Could you check a few things on this model? Use its own coordinates, in mm. Face numbers are marked on the shaded views. A direction names the side the tool comes from. Round coordinates to 2 decimals unless told otherwise and drop trailing zeros. Write each loop counter-clockwise with the first axis right and the second up, starting at its lowest first coordinate (ties: lowest second). Pieces come first, ordered by that corner, then holes. Notation, with made-up numbers: (62, 66) -> (121, 66) arc R35 ccw to (121, 101) -> close; hole circle Ø1 at (-29, -9.5). An arc over 180 degrees is marked (long way). Return JSON: item names as keys, results as strings.
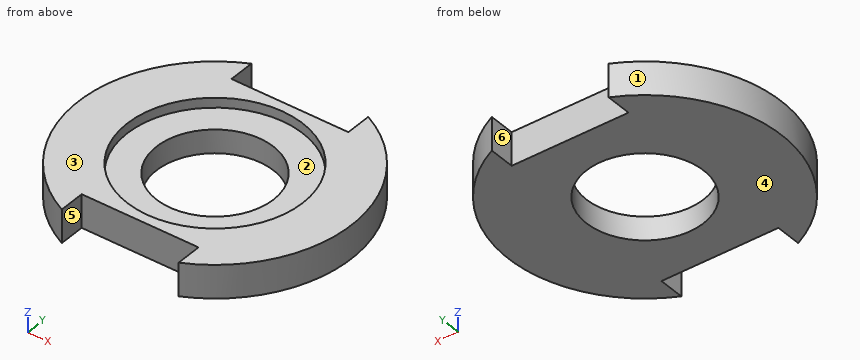
from build123d import *

# Parameters (mm, degrees)
SKETCH_1_R          = 14
EXTRUDE_1_DEPTH     = 3.4
SKETCH_2_R          = 6
CUT_EXTRUDE_1_DEPTH = 3.4
SKETCH_3_W          = 12
SKETCH_3_H          = 8
CUT_EXTRUDE_2_DEPTH = 3.4
SKETCH_4_R          = 9
CUT_EXTRUDE_3_DEPTH = 1


with BuildPart() as part:
    # 스케치1 → 보스-돌출1 (new body)
    with BuildSketch(Plane.XY):
        Circle(SKETCH_1_R)
    extrude(amount=EXTRUDE_1_DEPTH)

    # 스케치2 → 컷-돌출1 (cut)
    with BuildSketch(Plane.XY.offset(3.4)):
        Circle(SKETCH_2_R)
    extrude(amount=-CUT_EXTRUDE_1_DEPTH, mode=Mode.SUBTRACT)

    # 스케치3 → 컷-돌출2 (cut)
    with BuildSketch(Plane.XY.offset(3.4)):
        with Locations((0, 14)):
            Rectangle(SKETCH_3_W, SKETCH_3_H)
        with Locations((0, -14)):
            Rectangle(SKETCH_3_W, SKETCH_3_H)
    extrude(amount=-CUT_EXTRUDE_2_DEPTH, mode=Mode.SUBTRACT)

    # 스케치4 → 컷-돌출3 (cut)
    with BuildSketch(Plane.XY.offset(3.4)):
        Circle(SKETCH_4_R)
    extrude(amount=-CUT_EXTRUDE_3_DEPTH, mode=Mode.SUBTRACT)


solid = part.part
1) If I drill on probe 1 along Y at (x, z) = (0, 1.05); probe 2 along Y at (x, z) = (0, 2.9); probe 3 along Z at (x, y) = (-5.75, -5.75), over which ranges is the centre line in solid material (lowest first)? Write a range as [from, to].
Return value:
{"probe 1": "[-10, -6], [6, 10]", "probe 2": "[-10, -9], [9, 10]", "probe 3": "[0, 2.4]"}
2) I want a section at A-A, the plane x = 0. Please give me the cut outline in (y, z), and give its area (3 significant figures).
Return value:
{"outline": "(-10, 0) -> (-6, 0) -> (-6, 2.4) -> (-9, 2.4) -> (-9, 3.4) -> (-10, 3.4) -> close; (6, 0) -> (10, 0) -> (10, 3.4) -> (9, 3.4) -> (9, 2.4) -> (6, 2.4) -> close", "area": "21.2 mm²"}
3) I want a section at D-D, the plane y = -7. Please give me the cut outline in (x, z).
Return value:
{"outline": "(-12.12, 0) -> (12.12, 0) -> (12.12, 3.4) -> (5.66, 3.4) -> (5.66, 2.4) -> (-5.66, 2.4) -> (-5.66, 3.4) -> (-12.12, 3.4) -> close"}
4) I want a section at B-B, the plane z = 2.95. Please give me the cut outline in (x, y), and give its area (3 significant figures).
Return value:
{"outline": "(-6, -12.65) -> (-6, -10) -> (6, -10) -> (6, -12.65) arc R14 ccw to (6, 12.65) -> (6, 10) -> (-6, 10) -> (-6, 12.65) arc R14 ccw to start; hole circle Ø18 at (0, 0)", "area": "276 mm²"}
5) I want a section at C-C, the plane y = 0. Please give me the cut outline in (x, z), and give its area (3 significant figures).
Return value:
{"outline": "(-14, 0) -> (-6, 0) -> (-6, 2.4) -> (-9, 2.4) -> (-9, 3.4) -> (-14, 3.4) -> close; (6, 0) -> (14, 0) -> (14, 3.4) -> (9, 3.4) -> (9, 2.4) -> (6, 2.4) -> close", "area": "48.4 mm²"}
6) For the marked faces 4, 5 and 6, which set-ups out of +Z, -Z, +X, -X, +Y, -Y let a thin tool reach every point of the face, with its end or its side?
Return value:
{"face 4": "-Z, +X, -X, +Y, -Y", "face 5": "+Z, -Z, -Y", "face 6": "+Z, -Z, +Y"}
7) Thinking about a two-plate mould opening in Y: for the marked faces 1, 2 and 3, which applies, pulls with the +Y half, pulls with the -Y half, needs draft (parallel to the pull), parting line crosses it, or undercut?
Return value:
{"face 1": "parting line crosses it", "face 2": "undercut", "face 3": "needs draft"}
8) Will these pins go through, and if not, where does the flat tip stop? pin 1 Ø1.3 at (y, z) = (-10.5, 1.5) entering from -X; pin 2 Ø7 at (x, y) = (0, 0) entering from +Z; pin 3 Ø1 at (x, z) = (-7, 1.5) entering from -Y; pin 4 Ø14.5 at (x, y) = (0, -1.5) entering from +Z.
Return value:
{"pin 1": "x = -9.95", "pin 2": "through", "pin 3": "y = -12.4", "pin 4": "z = 2.4"}
